CAD build for the part. Positions are in the model's coordinates, mm. Face numbers are marked on the shaded views. A direction names the side the tool comes from. Round coordinates to 2 decimals unless told otherwise and drop trailing zeros. Loops run counter-clockwise (first coordinate to the right, second up) from the corner with the lowest first, then second, coordinate; pieces in that order, holes last.
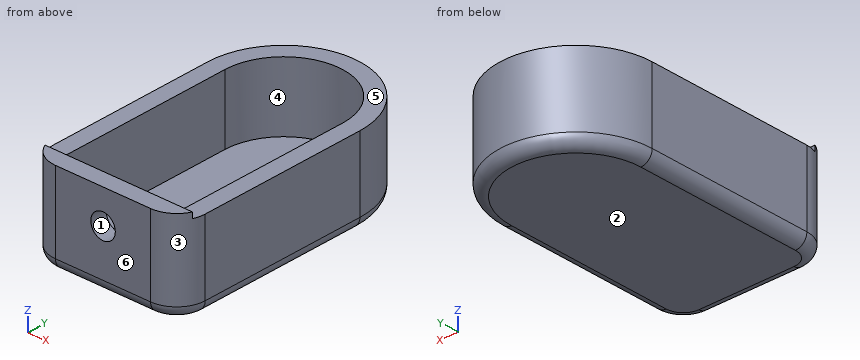
```python
from build123d import *

# Parameters (mm, degrees)
F1_DEPTH    = 3
F2_DEPTH    = 11.9
F4_DEPTH    = 1
F6_DEPTH    = 6
F7_T1_DEPTH = 40.9
F8_R        = 2
F9_R        = 3.5272638361
F10_DEPTH   = 1
F11_DEPTH   = 25


# Not quite as in the source:
# - a fillet or chamfer that OpenCascade refuses, or shapes differently, is made with other operations: its cross-section is extruded or revolved along the edge and cut away or added


with BuildPart() as f1:
    # F0 (on Top) → F1 (new body)
    with BuildSketch(Plane.XY):
        with BuildLine():
            Line((13.35, -34.6), (13.35, 0))
            ThreePointArc((13.35, 0), (0, 13.35), (-13.35, 0))
            Line((-13.35, 0), (-13.35, -34.6))
            Line((-13.35, -34.6), (13.35, -34.6))
        make_face()
        with BuildLine():
            Line((-10.35, -31.6), (-10.35, 0))
            ThreePointArc((-10.35, 0), (0, 10.35), (10.35, 0))
            Line((10.35, 0), (10.35, -31.6))
            Line((10.35, -31.6), (-10.35, -31.6))
        make_face(mode=Mode.SUBTRACT)
        with BuildLine():
            ThreePointArc((10.35, 0), (0, 10.35), (-10.35, 0))
            Line((-10.35, 0), (-10.35, -31.6))
            Line((-10.35, -31.6), (10.35, -31.6))
            Line((10.35, -31.6), (10.35, 0))
        make_face()
    extrude(amount=-F1_DEPTH)

    # F0 (on Top) → F2 (join)
    with BuildSketch(Plane.XY):
        with BuildLine():
            Line((13.35, -34.6), (13.35, 0))
            ThreePointArc((13.35, 0), (0, 13.35), (-13.35, 0))
            Line((-13.35, 0), (-13.35, -34.6))
            Line((-13.35, -34.6), (13.35, -34.6))
        make_face()
        with BuildLine():
            Line((-10.35, -31.6), (-10.35, 0))
            ThreePointArc((-10.35, 0), (0, 10.35), (10.35, 0))
            Line((10.35, 0), (10.35, -31.6))
            Line((10.35, -31.6), (-10.35, -31.6))
        make_face(mode=Mode.SUBTRACT)
    extrude(amount=F2_DEPTH)

    # F3 (on face) → F4 (join)
    with BuildSketch(Plane.XY.offset(11.9)):
        Polygon((-13.35, -34.6), (13.35, -34.6), (13.35, -31.6), (10.35, -31.6), (-10.35, -31.6), (-13.35, -31.6), align=None)
    extrude(amount=F4_DEPTH)

    # F5 (on face) → F6 (cut)
    with BuildSketch(Plane.XZ.offset(34.6)):
        with BuildLine():
            ThreePointArc((0, 9.2), (-2.15, 7.05), (0, 4.9))
            Line((0, 4.9), (0, 9.2))
        make_face()
        with BuildLine():
            Line((0, 9.2), (0, 4.9))
            ThreePointArc((0, 4.9), (1.5202795796, 5.5297204204), (2.15, 7.05))
            ThreePointArc((2.15, 7.05), (1.5202795796, 8.5702795796), (0, 9.2))
        make_face()
    extrude(amount=-F6_DEPTH, mode=Mode.SUBTRACT)

    # F7: fillet of radius 5 on 2 edges, made by hand

    # F7_s2 → F7_t1 (cut)
    with BuildSketch(Plane.XY.offset(-15.5)):
        with BuildLine():
            ThreePointArc((-13.35, -29.6), (-11.8855339059, -33.1355339059), (-8.35, -34.6))
            Line((-8.35, -34.6), (-13.35, -34.6))
            Line((-13.35, -34.6), (-13.35, -29.6))
        make_face()
        with BuildLine():
            ThreePointArc((8.35, -34.6), (11.8855339059, -33.1355339059), (13.35, -29.6))
            Line((13.35, -29.6), (13.35, -34.6))
            Line((13.35, -34.6), (8.35, -34.6))
        make_face()
    extrude(amount=F7_T1_DEPTH, mode=Mode.SUBTRACT)

    # F8
    f8_edges = [f1.edges().sort_by_distance(p)[0] for p in [
        (13.35, -14.8, -3),
    ]]
    fillet(f8_edges, radius=F8_R)

    # F9 (on face) → F10 (join)
    with BuildSketch(Plane(origin=(0, -31.6, 0), x_dir=(-1, 0, 0), z_dir=(0, 1, 0))):
        with Locations((0, 7.05)):
            Circle(F9_R)
    extrude(amount=-F10_DEPTH)

    # F11 (cut): a face of the model
    f11_faces = [f1.faces().sort_by_distance(p)[0] for p in [
        (0, -32.6, 7.05),
    ]]
    extrude(f11_faces, amount=-F11_DEPTH, mode=Mode.SUBTRACT)


solid = f1.part
```
Item 1: Cut at B-B, the plane z = 2. Give the cut face in (x, y).
Answers follow:
outline: (-13.35, -29.6) arc R5 ccw to (-8.35, -34.6) - (8.35, -34.6) arc R5 ccw to (13.35, -29.6) - (13.35, 0) arc R13.35 ccw to (-13.35, 0) - close; hole (-10.35, -31.6) - (10.35, -31.6) - (10.35, 0) arc R10.35 ccw to (-10.35, 0) - close
Item 2: Cut at A-A, the plane x = 0. Give the cut face in (y, z).
Answers follow:
outline: (-34.6, -1) arc R2 ccw to (-32.6, -3) - (11.35, -3) arc R2 ccw to (13.35, -1) - (13.35, 11.9) - (10.35, 11.9) - (10.35, 0) - (-31.6, 0) - (-31.6, 4.9) - (-34.6, 4.9) - close; (-34.6, 9.2) - (-31.6, 9.2) - (-31.6, 12.9) - (-34.6, 12.9) - close
Item 3: Cut at D-D, the plane z = 7.05. Give the cut face in (x, y).
Answers follow:
outline: (-13.35, -29.6) arc R5 ccw to (-8.35, -34.6) - (-2.15, -34.6) - (-2.15, -31.6) - (-10.35, -31.6) - (-10.35, 0) arc R10.35 cw to (10.35, 0) - (10.35, -31.6) - (2.15, -31.6) - (2.15, -34.6) - (8.35, -34.6) arc R5 ccw to (13.35, -29.6) - (13.35, 0) arc R13.35 ccw to (-13.35, 0) - close
Item 4: Probe line 1 (X direction, y = -13.5, z = 2.5); line 2 (X direction, y = -33.6, z = 7.05); line 3 (Y direction, x = 0, z = 7.75). List the from-to ranges inside material, lowest first.
Answers follow:
line 1: x = -13.35 to -10.35, 10.35 to 13.35
line 2: x = -11.35 to -2.15, 2.15 to 11.35
line 3: y = 10.35 to 13.35
Item 5: Cut at C-C, the plane y = -21.5. Give the cut face in (x, z).
Answers follow:
outline: (-13.35, -1) arc R2 ccw to (-11.35, -3) - (11.35, -3) arc R2 ccw to (13.35, -1) - (13.35, 11.9) - (10.35, 11.9) - (10.35, 0) - (-10.35, 0) - (-10.35, 11.9) - (-13.35, 11.9) - close
Item 6: Flat gauge pins, fed straight in: P1, Ø1, axis at x = 7, y = -28, coming from the +Z side; P2, Ø1.5, axis at x = -10, z = 10.5, coming from the +Y side. Where does each tip first touch, or does it go through?
Answers follow:
P1: stops at z = 0
P2: stops at y = 9.63
Item 7: 3-axis set-ups, long thin cutter, end or side, ignore diameter. For the marked faces 4, 5 and 6: which of +Z, -Z, +X, -X, +Y, -Y reach the whole face in a straight line?
Answers follow:
face 4: +Z
face 5: +Z, +X, -X, +Y
face 6: +Z, -Z, +X, -X, -Y
Item 8: Two-plate mould, pull along X, no slides. Class the marked faces 1, 2 and 3: released by +X, released by -X, zero draft, split by the parting line, or undercut.
Answers follow:
face 1: undercut
face 2: zero draft
face 3: released by +X
